Design review of the part built by this model. Coordinates are the model's own, in mm. Face numbers are marked on the shaded views. A direction names the side the tool comes from. Round coordinates to 2 decimals unless told otherwise and drop trailing zeros. Order: outer loops, then holes, each group sorted by start corner. A loop starts at its lowest first (then second) coordinate and runs counter-clockwise, first axis right, second up. Notation, with made-up numbers: M -16.75,74 L 36.25,74 A26 ccw 36.25,91 Z; hole C 33,59.25 d10. An arc over 180 degrees is marked long. Use a Markdown table: item, result. Add a question column.
(1) Take a section at B-B (z = 0). Write out the cut boundary in (x, y).
(2) For pin 1 (4 mm diameter, centred on x = 62.5, y = -1.5, fed in from -Z); pin 2 (6 mm diameter, centred on x = 51, y = 5.5, fed in from -Z); pin 3 (1 mm diameter, centred on y = -7.5, z = -3, fed in from -X); pin 4 (8.5 mm diameter, centred on x = 140, z = 0, fed in from +Y), all flat-tipped, find the tip position at first contact; note any pin that passes through.
(3) Take a section at C-C (y = -0.75). Write out the cut boundary in (x, z).
(4) To check wall thickness, follow probe 1 along X at (y, z) = (3.25, 0); probe 2 along Z at (x, y) = (0, 3.25); probe 3 along Z at (x, y) = (-12, 3). State the ranges of each line that lie inside material, in increasing order. Write a range as from..to.
(5) The part is to be moulded in two halves that separate along X. For the marked faces 1, 2 and 3, say which applies: released by +X, released by -X, zero draft, split by the parting line, or undercut.
(6) Take a section at D-D (x = -5). Write out the cut boundary in (y, z).
(7) Machinability: for the marked faces 4, 5, 6 and 7, which of the approach directions +Z, -Z, +X, -X, +Y, -Y give a long, thin tool a straight path to every point of the face, cutting with its end or side? Answer none if there is none.
(8) Take a section at A-A (x = 140). Write out the cut boundary in (y, z).
```python
from build123d import *

# Parameters (mm, degrees)
SKETCH1_R           = 30
SKETCH1_R_2         = 7
BOSS_EXTRUDE1_DEPTH = 10
FILLET1_R           = 20
FILLET2_R           = 10
CUT_EXTRUDE1_DEPTH  = 21


with BuildPart() as part:
    # Sketch1 → Boss-Extrude1 (new body, symmetric)
    with BuildSketch(Plane(origin=(0, 0, 0), x_dir=(1, 0, 0), z_dir=(0, 1, 0))):
        with BuildLine():
            Line((27.935473676, 25.760615491), (128.063755469, 9.084385863))
            ThreePointArc((128.063755469, 9.084385863), (155, 0), (128.063755469, -9.084385863))
            Line((128.063755469, -9.084385863), (27.935473676, -25.760615491))
            ThreePointArc((27.935473676, -25.760615491), (-38, 0), (27.935473676, 25.760615491))
        make_face()
        Circle(SKETCH1_R, mode=Mode.SUBTRACT)
        with Locations((140, 0)):
            Circle(SKETCH1_R_2, mode=Mode.SUBTRACT)
    extrude(amount=BOSS_EXTRUDE1_DEPTH, both=True)

    # Fillet1
    fillet1_edges = [part.edges().sort_by_distance(p)[0] for p in [
        (27.935473676, 0, -25.760615491),
        (27.935473676, 0, 25.760615491),
    ]]
    fillet(fillet1_edges, radius=FILLET1_R)

    # Fillet2
    fillet2_edges = [part.edges().sort_by_distance(p)[0] for p in [
        (128.063755469, 0, -9.084385863),
        (128.063755469, 0, 9.084385863),
    ]]
    fillet(fillet2_edges, radius=FILLET2_R)

    # Sketch2 → Cut-Extrude1 (cut, through all)
    with BuildSketch(Plane(origin=(0, 10, 0), x_dir=(1, 0, 0), z_dir=(0, 1, 0))):
        with BuildLine():
            Line((41.828554558, 17.870982725), (122.478416149, 4.438857582))
            ThreePointArc((122.478416149, 4.438857582), (126.239130435, 0), (122.478416149, -4.438857582))
            Line((122.478416149, -4.438857582), (41.828554558, -17.870982725))
            ThreePointArc((41.828554558, -17.870982725), (37.231968897, -16.217361812), (36.238855523, -11.43439331))
            ThreePointArc((36.238855523, -11.43439331), (38, 0), (36.238855523, 11.43439331))
            ThreePointArc((36.238855523, 11.43439331), (37.231968897, 16.217361812), (41.828554558, 17.870982725))
        make_face()
    extrude(amount=-CUT_EXTRUDE1_DEPTH, mode=Mode.SUBTRACT)


solid = part.part
```
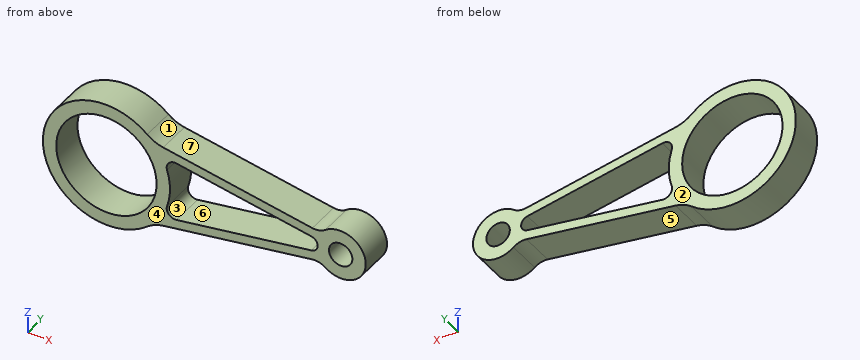
Verdict:
| question | item | result |
|---|---|---|
| 1 | outline | M -38,-10 L -30,-10 L -30,10 L -38,10 Z; M 30,-10 L 38,-10 L 38,10 L 30,10 Z; M 126.24,-10 L 133,-10 L 133,10 L 126.24,10 Z; M 147,-10 L 155,-10 L 155,10 L 147,10 Z |
| 2 | pin 1 | stops at z = -20.34 |
| 2 | pin 2 | stops at z = -22.42 |
| 2 | pin 3 | stops at x = -37.92 |
| 2 | pin 4 | passes through |
| 3 | outline | M 24.38,-29.15 A20 cw 33.92,-24.76 L 123.07,-9.92 A10 cw 130.83,-11.87 A15 ccw long 130.83,11.87 A10 cw 123.07,9.92 L 33.92,24.76 A20 cw 24.38,29.15 A38 ccw long Z; hole C 0,0 d60; hole M 36.24,-11.43 A5 ccw 41.83,-17.87 L 122.48,-4.44 A4.5 ccw 122.48,4.44 L 41.83,17.87 A5 ccw 36.24,11.43 A38 cw Z; hole C 140,0 d14 |
| 4 | probe 1 | x = -38..-30, 30..38, 126.24..133, 147..155 |
| 4 | probe 2 | z = -38..-30, 30..38 |
| 4 | probe 3 | z = -36.06..-27.5, 27.5..36.06 |
| 5 | face 1 | released by +X |
| 5 | face 2 | zero draft |
| 5 | face 3 | undercut |
| 6 | outline | M -10,-37.67 L 10,-37.67 L 10,-29.58 L -10,-29.58 Z; M -10,29.58 L 10,29.58 L 10,37.67 L -10,37.67 Z |
| 7 | face 4 | +Z, -Z, +X, -X, -Y |
| 7 | face 5 | -Z, +Y, -Y |
| 7 | face 6 | +Y, -Y |
| 7 | face 7 | +Z, +Y, -Y |
| 8 | outline | M -10,-15 L 10,-15 L 10,-7 L -10,-7 Z; M -10,7 L 10,7 L 10,15 L -10,15 Z |
